Source: three-view drawing plus pictorial views. Frame: mm from the lowest corner of the part. Coordinates: 2 decimals unless noted, no trailing zeros. Write each loop counter-clockwise with the first axis right and the second up, starting at its lowest first coordinate (ties: lowest second). Pieces come first, ordered by that corner, then holes. Notation, with made-up numbers: M -18,16.25 L 3,16.25 A27 cw 3,55.25 Z; hole C 46,72 d3. An arc over 180 degrees is marked long. Write item = value, one per line. Start each with the question number.
Item 1: First-contact query: pin 1 Ø3.5 at (y, z) = (3, 11) entering from +X. Flat tip, straight axial feed; report the tip coordinate or a pass-through.
Item 2: Pull-direction query (Z, two-part tool) for the marked faces 1, 2 and 3; classes: +Z half, -Z half, draft (parallel to the pull), parting line (faces both ways), or undercut.
Item 3: Section A-A on z = 3. Output: boundary loops of the cut face in (x, y).
Item 4: Section C-C on y = 3. Give the number of separate pieces and of enclosed holes in the cut face.
Item 5: Section D-D on y = 0.75. Output: boundary loops of the cut face in (x, z).
Item 6: Ray query, L1, parallel to Z at x = 0.1, y = 2 (1 decimal); L2, parallel to Z at x = 0.7, y = 1.75; L3, parallel to Y at x = 0.65, z = 11. Return the intervals inside material, ascending. Write a range as [from, to].
Item 7: Section B-B on x = 1.2. Output: boundary loops of the cut face in (y, z) (1 decimal).
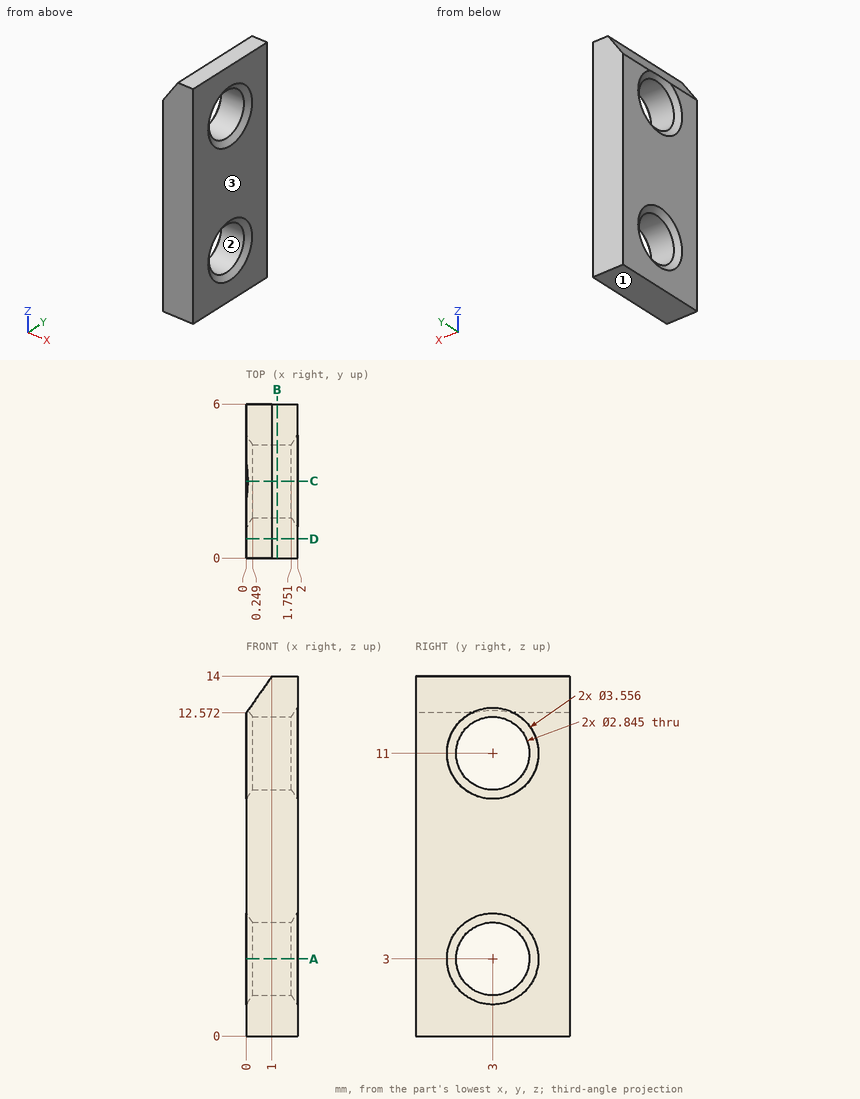
Responses:
q1.pin_1 = 1.98
q2.face_1 = -Z half
q2.face_2 = undercut
q2.face_3 = draft
q3.outline = M 0,0 L 2,0 L 2,1.22 L 1.75,1.58 L 0.25,1.58 L 0,1.22 Z; M 0,4.78 L 0.25,4.42 L 1.75,4.42 L 2,4.78 L 2,6 L 0,6 Z
q4.separate_pieces = 3
q4.enclosed_holes = 0
q5.outline = M 0,0 L 2,0 L 2,14 L 1,14 L 0,12.57 Z
q6.L1 = [0, 1.7], [4.3, 9.7], [12.3, 12.7]
q6.L2 = [0, 2.32], [3.68, 10.32], [11.68, 13.57]
q6.L3 = [0, 1.58], [4.42, 6]
q7.outline = M 0,0 L 6,0 L 6,14 L 0,14 Z; hole C 3,3 d2.8; hole C 3,11 d2.8
